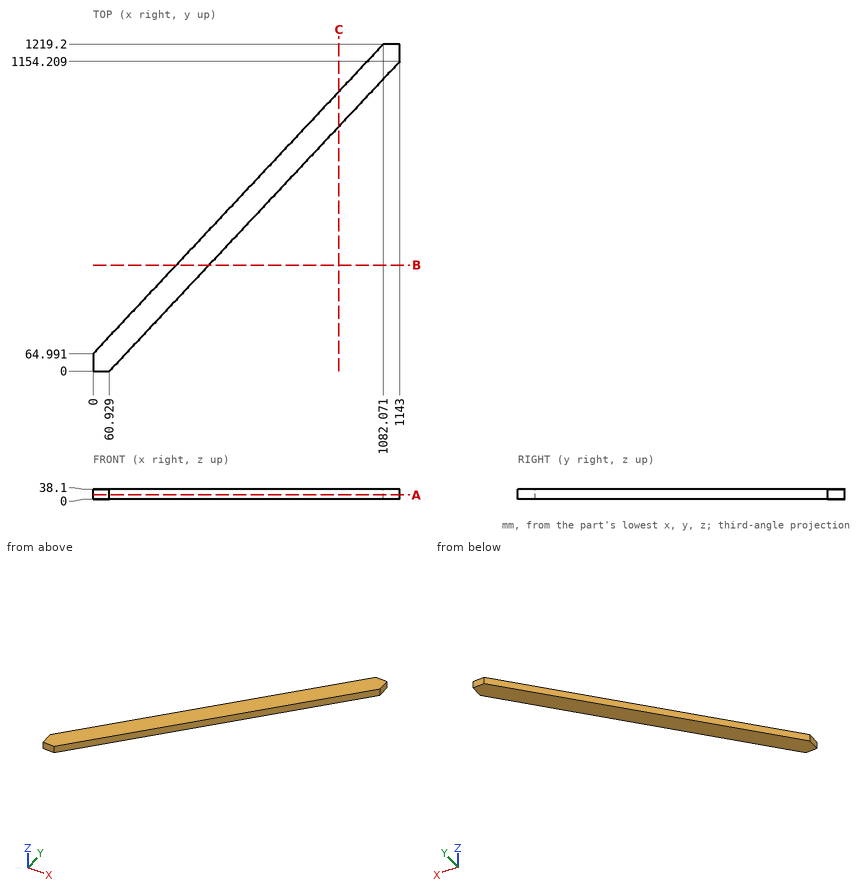
Print and shaded views of the part. All mm, measured from the part's lowest x, y and z. Coordinates: 2 decimals unless noted, no trailing zeros. Order: outer loops, then holes, each group sorted by start corner. A loop starts at its lowest first (then second) coordinate and runs counter-clockwise, first axis right, second up. Notation, with made-up numbers: (50, 41.25) - (87, 41.25) arc R16 ccw to (87, 45.25) - close; hole circle Ø7 at (75.25, 2.25). An arc over 180 degrees is marked (long way). Put each result on its own line as item: value.
1. Drop flat-ended pins along their axis: P1, Ø1, axis at y = 138.5, z = 17.5, coming from the +X side; P2, Ø10, axis at x = 605.5, z = 30, coming from the +Y side; P3, Ø12, axis at y = 1097, z = 30.5, coming from the +X side. Give the stop position or say it passes through.
Answer sheet:
P1: stops at x = 191.24
P2: stops at y = 716.19
P3: stops at x = 1094.99
2. Saw through at A-A (z = 17.5). Write the cut outline in (x, y).
Answer sheet:
outline: (0, 0) - (60.93, 0) - (1143, 1154.21) - (1143, 1219.2) - (1082.07, 1219.2) - (0, 64.99) - close
3. Probe line 1 along Y through (x, z) = (990, 23); line 2 along X through (y, z) = (703, 7); line 3 along X through (y, z) = (1122.5, 19). List the from-to ranges inside material, lowest first. Write a range as [from, to].
Answer sheet:
line 1: y = [991.01, 1120.99]
line 2: x = [598.13, 719.99]
line 3: x = [991.41, 1113.27]
4. Saw through at C-C (x = 916.5). Write the cut outline in (y, z).
Answer sheet:
outline: (912.61, 0) - (1042.59, 0) - (1042.59, 38.1) - (912.61, 38.1) - close
5. Saw through at B-B (y = 395). Write the cut outline in (x, z).
Answer sheet:
outline: (309.38, 0) - (431.24, 0) - (431.24, 38.1) - (309.38, 38.1) - close
